from build123d import *

# Parameters (mm, degrees)
SKETCH_1_R          = 1.5
EXTRUDE_1_DEPTH     = 5
SKETCH_2_R          = 3
CUT_EXTRUDE_1_DEPTH = 10


with BuildPart() as part:
    # 草图1 → 凸台-拉伸1 (new body)
    with BuildSketch(Plane.XY):
        with BuildLine():
            Line((-15.5, 27.5), (38.5, 27.5))
            ThreePointArc((38.5, 27.5), (40.621320344, 26.621320344), (41.5, 24.5))
            Line((41.5, 24.5), (41.5, -7))
            ThreePointArc((41.5, -7), (40.621320344, -9.121320344), (38.5, -10))
            Line((38.5, -10), (33.3, -10))
            Line((33.3, -10), (30.825, -10))
            Line((30.825, -10), (30.825, 10))
            Line((30.825, 10), (-9.175, 10))
            Line((-9.175, 10), (-9.175, -10))
            Line((-9.175, -10), (-15.5, -10))
            ThreePointArc((-15.5, -10), (-17.621320344, -9.121320344), (-18.5, -7))
            Line((-18.5, -7), (-18.5, 24.5))
            ThreePointArc((-18.5, 24.5), (-17.621320344, 26.621320344), (-15.5, 27.5))
        make_face()
        with Locations((-13.575, 5)):
            Circle(SKETCH_1_R, mode=Mode.SUBTRACT)
        with Locations((-13.575, -5)):
            Circle(SKETCH_1_R, mode=Mode.SUBTRACT)
        with Locations((35.025, 5)):
            Circle(SKETCH_1_R, mode=Mode.SUBTRACT)
        with Locations((35.025, -5)):
            Circle(SKETCH_1_R, mode=Mode.SUBTRACT)
    extrude(amount=EXTRUDE_1_DEPTH)

    # 草图2 → 切除-拉伸1 (cut)
    with BuildSketch(Plane.XY.offset(5)):
        with Locations((-6.17, 21.5)):
            Circle(SKETCH_2_R)
        with Locations((29.17, 21.5)):
            Circle(SKETCH_2_R)
    extrude(amount=-CUT_EXTRUDE_1_DEPTH, mode=Mode.SUBTRACT)


solid = part.part
Source: CAD feature listing. Evaluate the final solid. Frame: model axes, mm. A direction names the side the tool comes from. Coordinates: 2 decimals unless noted, no trailing zeros. Loops run counter-clockwise (first coordinate to the right, second up) from the corner with the lowest first, then second, coordinate; pieces in that order, holes last. Notation, with made-up numbers: (-33, 42) - (7, 42) arc R9 ccw to (7, 51) - close; hole circle Ø5 at (60.25, 75.25). An arc over 180 degrees is marked (long way). One line per question, with ' | ' between items.
1) Section B-B, the plane y = 2.5. Return loops of the section in (x, z) (3 decimals).
Report:
outline: (-18.5, 0) - (-9.175, 0) - (-9.175, 5) - (-18.5, 5) - close; (30.825, 0) - (41.5, 0) - (41.5, 5) - (30.825, 5) - close
2) Section D-D, the plane y = -5. Return loops of the section in (x, z) (3 decimals), then the cut area to 3 significant figures.
Report:
outline: (-18.5, 0) - (-15.075, 0) - (-15.075, 5) - (-18.5, 5) - close; (-12.075, 0) - (-9.175, 0) - (-9.175, 5) - (-12.075, 5) - close; (30.825, 0) - (33.525, 0) - (33.525, 5) - (30.825, 5) - close; (36.525, 0) - (41.5, 0) - (41.5, 5) - (36.525, 5) - close | area: 70.0 mm²
3) Section A-A, the plane x = -6.17. Return loops of the section in (y, z), then the cut area to 3 significant figures.
Report:
outline: (10, 0) - (18.5, 0) - (18.5, 5) - (10, 5) - close; (24.5, 0) - (27.5, 0) - (27.5, 5) - (24.5, 5) - close | area: 57.5 mm²
4) Section C-C, the plane z = 3.15. Return loops of the section in (x, y) (3 decimals), then the cut area to 3 significant figures.
Report:
outline: (-18.5, -7) arc R3 ccw to (-15.5, -10) - (-9.175, -10) - (-9.175, 10) - (30.825, 10) - (30.825, -10) - (38.5, -10) arc R3 ccw to (41.5, -7) - (41.5, 24.5) arc R3 ccw to (38.5, 27.5) - (-15.5, 27.5) arc R3 ccw to (-18.5, 24.5) - close; hole circle Ø3 at (-13.575, -5); hole circle Ø3 at (-13.575, 5); hole circle Ø6 at (-6.17, 21.5); hole circle Ø6 at (29.17, 21.5); hole circle Ø3 at (35.025, -5); hole circle Ø3 at (35.025, 5) | area: 1,360 mm²
5) Line query: line 1 along Y through (x, z) = (35, 1.9); line 2 along X through (y, z) = (-2, 3.2) (3 decimals); line 3 along X through (y, z) = (20, 2.65). Output: solid intervals per line, ascending.
Report:
line 1: y = -10 to -6.5, -3.5 to 3.5, 6.5 to 27.5 | line 2: x = -18.5 to -9.175, 30.825 to 41.5 | line 3: x = -18.5 to -8.77, -3.57 to 26.57, 31.77 to 41.5
6) First-contact query: P1, Ø2.5, axis at x = 35.025, y = 5, coming from the -Z side; P2, Ø2, axis at x = 8, z = 2, coming from the -Y side. Flat tips, straight axial feed; report the tip coordinate or a pass-through.
Report:
P1: passes through | P2: stops at y = 10
7) Set-up query: faces 1 (the face through (11, 10, 2)), 2 (the face through (12, 13, 0)). Return all of +Z, -Z, +X, -X, +Y, -Y with unobstructed straight access to the full face (end or side cutting, diameter ignored); none if empty.
Report:
face 1: +Z, -Z, -Y | face 2: -Z, +X, -X, +Y, -Y
8) Pull-direction query (X, two-part tool) for faces 3 (the face through (30.825, 0, 2)), 4 (the face through (-18.5, 9, 2)), 5 (the face through (41.5, 9, 2)); classes: released by +X, released by -X, zero draft, split by the parting line, or undercut.
Report:
face 3: undercut | face 4: released by -X | face 5: released by +X
